```python
from build123d import *

# Parameters (mm, degrees)
SKETCH_1_R          = 3
EXTRUDE_1_DEPTH     = 40
SKETCH_2_R          = 1.427663882
CUT_EXTRUDE_1_DEPTH = 41.224370722
CHAMFER_1_SIZE      = 1


with BuildPart() as part:
    # 草图1 → 凸台-拉伸1 (new body)
    with BuildSketch(Plane(origin=(0, 0, 0), x_dir=(1, 0, 0), z_dir=(0, 1, 0))):
        with Locations(Location((0, 0, 0), (0, 0, 270))):
            Circle(SKETCH_1_R)
    extrude(amount=EXTRUDE_1_DEPTH)

    # 草图2 → 切除-拉伸1 (cut, through all)
    with BuildSketch(Plane.XZ):
        with Locations(Location((0, 0, 0), (0, 0, 270))):
            Circle(SKETCH_2_R)
    extrude(amount=-CUT_EXTRUDE_1_DEPTH, mode=Mode.SUBTRACT)

    # 倒角1
    chamfer_1_edges = [part.edges().sort_by_distance(p)[0] for p in [
        (0, 0, -3),
    ]]
    chamfer(chamfer_1_edges, length=CHAMFER_1_SIZE)


solid = part.part
```
Geometry check sheet. Reference: the model listing, model coordinates, mm. Coordinates: 2 decimals unless noted, no trailing zeros. Order: outer loops, then holes, each group sorted by start corner. A loop starts at its lowest first (then second) coordinate and runs counter-clockwise, first axis right, second up. Notation, with made-up numbers: (23.25, 41.25) - (54.25, 41.25) arc R27 ccw to (54.25, 73.25) - close; hole circle Ø11 at (-13, 36). An arc over 180 degrees is marked (long way). Use one line per item in the form item = value.
1. Section check A-A (z = 0). Record the boundary of the cut face in (x, y).
Here are the results:
outline = (-3, 1) - (-2, 0) - (-1.43, 0) - (-1.43, 40) - (-3, 40) - close; (1.43, 0) - (2, 0) - (3, 1) - (3, 40) - (1.43, 40) - close
2. Scan lines: line 1 (X direction, y = 10.5, z = 0); line 2 (Z direction, x = 0.4, y = 37); line 3 (X direction, y = 19, z = 1.1). Record each from-to range of solid material in increasing order.
Here are the results:
line_1 = -3 to -1.43, 1.43 to 3
line_2 = -2.97 to -1.37, 1.37 to 2.97
line_3 = -2.79 to -0.91, 0.91 to 2.79
3. Draft check along X on faces 1 (the face through (-1.394, 19.72, 0.309)), 2 (the face through (-1.3, 0, 0.9)), 3 (the face through (0.9, 20.23, 2.86)). Enter one of: pulls with the +X half, pulls with the -X half, needs draft (parallel to the pull), parting line crosses it, or undercut.
Here are the results:
face_1 = undercut
face_2 = needs draft
face_3 = parting line crosses it
4. Section check B-B (x = 0). Record the boundary of the cut face in (y, z), then the cut area to 3 significant figures.
Here are the results:
outline = (0, -2) - (1, -3) - (40, -3) - (40, -1.43) - (0, -1.43) - close; (0, 1.43) - (40, 1.43) - (40, 3) - (1, 3) - (0, 2) - close
area = 125 mm²
5. Section check C-C (y = 15). Record the boundary of the cut face in (x, z).
Here are the results:
outline = circle Ø6 at (0, 0); hole circle Ø2.86 at (0, 0)
6. Gauge pin test, flat ends, axial feed: pin 1 (1.5 mm diameter, centred on y = 5, z = -1.5, fed in from +X); pin 2 (1.5 mm diameter, centred on y = 15, z = 2.5, fed in from +X). Record the tip position at first contact, or that the pin passes through.
Here are the results:
pin_1 = 2.9
pin_2 = 2.44
